Could you check a few things on this model? Use its own coordinates, in mm. A direction names the side the tool comes from. Round coordinates to 2 decimals unless told otherwise and drop trailing zeros. Order: outer loops, then holes, each group sorted by start corner. A loop starts at its lowest first (then second) coordinate and runs counter-clockwise, first axis right, second up. Notation, with made-up numbers: M -14.5,57 L 39.5,57 A17 cw 39.5,88 Z; hole C 32.25,65.25 d6. An arc over 180 degrees is marked long. Write each question's results on one line, items separated by ' | '. Start each with the question number.
1. For faces 1 (the cylindrical face through (-0.54, -2.44, 3.11)), 2 (the flat face through (0, 0, 0)), which set-ups out of +Z, -Z, +X, -X, +Y, -Y let a thin tool reach every point of the face, with its end or its side?
2. Suppose I cut it at A-A on x = 0. Write out the boundary of the cut face in (y, z).
3. Suppose I cut it at D-D on z = 7.75. Write out the boundary of the cut face in (x, y).
4. Please list where these lines run through material, in increasing order: L1, parallel to X at y = 0.1, z = 5; L2, parallel to X at y = 1.95, z = 7.25.
5. Suppose I cut it at C-C on z = 3.5. Write out the boundary of the cut face in (x, y), and give its area (3 significant figures).
6. I'm going to push flat-ended pins straight in: pin 1 (3 mm diameter, centred on y = -2, z = 2, fed in from -X); pin 2 (1.5 mm diameter, centred on y = 2, z = 5.5, fed in from -X). Where does each tip first touch, or does it pass through?
from build123d import *

# Parameters (mm, degrees)
F0_W     = 5.9
F0_H     = 5.9
F0_R     = 2.5
F1_DEPTH = 0.1
F2_DEPTH = 8.7
F3_R     = 2.5


with BuildPart() as f1:
    # F0 (on Top) → F1 (new body)
    with BuildSketch(Plane.XY):
        Rectangle(F0_W, F0_H)
        Circle(F0_R, mode=Mode.SUBTRACT)
    extrude(amount=F1_DEPTH)

    # F0 (on Top) → F2 (join)
    with BuildSketch(Plane.XY):
        Circle(F0_R)
    extrude(amount=F2_DEPTH)

    # F3
    f3_edges = [f1.edges().sort_by_distance(p)[0] for p in [
        (-2.5, 0, 8.7),
    ]]
    fillet(f3_edges, radius=F3_R)


solid = f1.part
Filled sheet:
1) face 1: +Z | face 2: -Z, +X, -X, +Y, -Y
2) outline: M -2.95,0 L 2.95,0 L 2.95,0.1 L 2.5,0.1 L 2.5,6.2 A2.5 ccw -2.5,6.2 L -2.5,0.1 L -2.95,0.1 Z
3) outline: C 0,0 d3.92
4) L1: x = -2.5 to 2.5 | L2: x = -1.16 to 1.16
5) outline: C 0,0 d5 | area: 19.6 mm^2
6) pin 1: stops at x = -2.45 | pin 2: stops at x = -2.17
